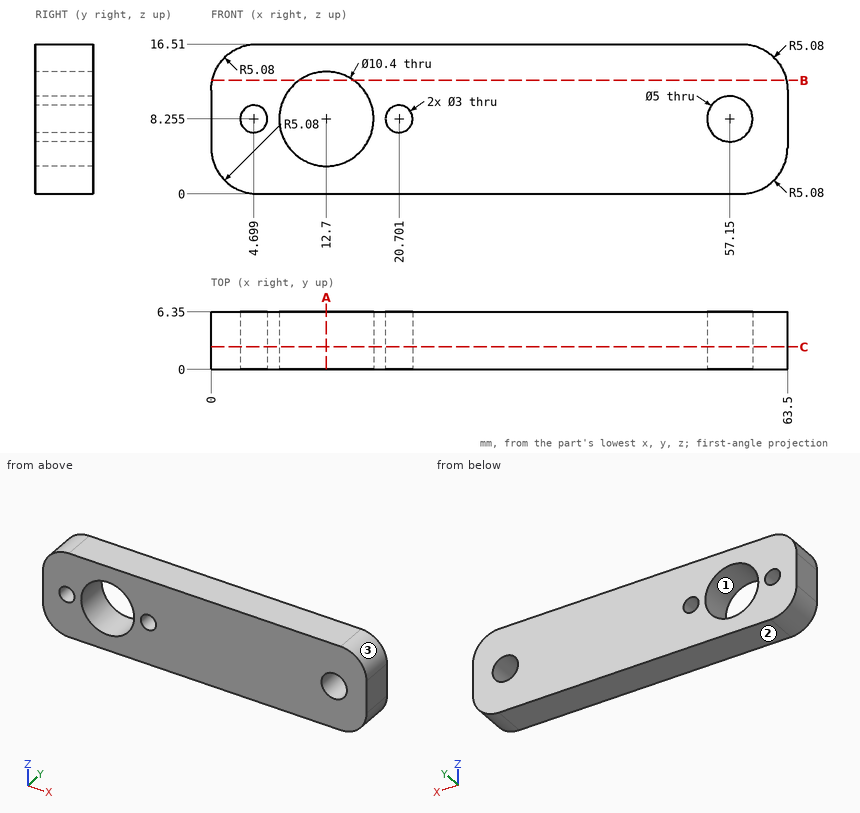
Input: dimensioned drawing with shaded views. Units: mm. Origin: part minimum x, y, z. Round coordinates to 2 decimals unless told otherwise and drop trailing zeros. Loops run counter-clockwise (first coordinate to the right, second up) from the corner with the lowest first, then second, coordinate; pieces in that order, holes last.
1) Pull-direction query (Z, two-part tool) for the marked faces 1, 2 and 3; classes: released by +Z, released by -Z, zero draft, split by the parting line, or undercut.
Ans:
face 1: undercut
face 2: released by -Z
face 3: released by +Z
2) Section query B-B on z = 12.5. Return the cut outline in (x, y), plus the area to 3 significant figures.
Ans:
outline: (0.11, 0) - (9.7, 0) - (9.7, 6.35) - (0.11, 6.35) - close; (15.7, 0) - (63.39, 0) - (63.39, 6.35) - (15.7, 6.35) - close
area: 364 mm2
3) Section query A-A on x = 12.7. Return the cut outline in (y, z) (3 decimals).
Ans:
outline: (0, 0) - (6.35, 0) - (6.35, 3.055) - (0, 3.055) - close; (0, 13.455) - (6.35, 13.455) - (6.35, 16.51) - (0, 16.51) - close
4) Pin query (flat end, axial travel): pin 1 (8 mm diameter, centred on x = 30.5, z = 3.5, fed in from -Y); pin 2 (1 mm diameter, centred on y = 4.5, z = 14, fed in from +X). Return the tip coordinate at first contact, or that it passes through.
Ans:
pin 1: stops at y = 0
pin 2: stops at x = 63.06
5) Material intervals for line 1 (Z direction, x = 13, y = 4); line 2 (Z direction, x = 57.15, y = 3.75) (3 decimals); line 3 (X direction, y = 6, z = 9), sorted ascending.
Ans:
line 1: z = 0 to 3.06, 13.45 to 16.51
line 2: z = 0 to 5.755, 10.755 to 16.51
line 3: x = 0 to 3.4, 6 to 7.55, 17.85 to 19.4, 22 to 54.76, 59.54 to 63.5
6) Section query C-C on y = 2.5. Return the cut outline in (x, z) (3 decimals), plus the area to 3 significant figures.
Ans:
outline: (0, 5.08) arc R5.08 ccw to (5.08, 0) - (58.42, 0) arc R5.08 ccw to (63.5, 5.08) - (63.5, 11.43) arc R5.08 ccw to (58.42, 16.51) - (5.08, 16.51) arc R5.08 ccw to (0, 11.43) - close; hole circle Ø3 at (4.699, 8.255); hole circle Ø10.4 at (12.7, 8.255); hole circle Ø3 at (20.701, 8.255); hole circle Ø5 at (57.15, 8.255)
area: 908 mm2
